from build123d import *

# Parameters (mm, degrees)
F0_R     = 3.81
F1_DEPTH = 25.4


with BuildPart() as f1:
    # F0 (on Top) → F1 (new body)
    with BuildSketch(Plane.XY):
        Polygon((-116.922736, 72.318586), (-370.922736, 72.318586), (-370.922736, 46.918586), (-256.622736, 48.152742), (-256.622736, 35.452742), (-243.922736, 35.452742), (-243.922736, 48.152742), (-129.622736, 48.152742), (-129.622736, 35.452742), (-116.922736, 35.452742), (-116.922736, 46.918586), align=None)
        with Locations((-250.272736, 41.802742)):
            Circle(F0_R, mode=Mode.SUBTRACT)
        with Locations((-122.94844, 41.478446)):
            Circle(F0_R, mode=Mode.SUBTRACT)
    extrude(amount=F1_DEPTH)


solid = f1.part
Can you work these out from the model? Positions are in its coordinate system, mm. A direction names the side the tool comes from. Coordinates: 2 decimals unless noted, no trailing zeros. Write each loop counter-clockwise with the first axis right and the second up, starting at its lowest first coordinate (ties: lowest second). Pieces come first, ordered by that corner, then holes. Notation, with made-up numbers: (74.5, -27.5) - (103.5, -27.5) arc R16 cw to (103.5, -13.5) - close; hole circle Ø3 at (60.25, -40). An arc over 180 degrees is marked (long way). Return JSON: item names as keys, results as strings. Group by question number.
Item 1: I'm going to push a flat-ended pin straight in: pin 1 Ø6.5 at (y, z) = (39, 13) entering from -X. Where does the tip first touch, or does it pass through?
Item 2: If we section it at C-C (x = -352.5): Write out the boundary of the cut face in (y, z).
Item 3: Please list where these lines run through material, in increasing order: probe 1 along X at (y, z) = (42, 15); probe 2 along X at (y, z) = (46, 23); probe 3 along Y at (x, z) = (-171, 19.25).
Item 4: If we section it at B-B (x = -137.5): Write out the boundary of the cut face in (y, z).
Item 5: We'd pull the mould along X, two halves only. Please class faces 1 (the face through (-129.623, 42, 13)), 2 (the face through (-116.923, 54, 13)), 3 (the face through (-242, 72.319, 13)): pulls with the +X half, pulls with the -X half, needs draft (parallel to the pull), parting line crosses it, or undercut.
Item 6: Which directions (+Z, -Z, +X, -X, +Y, -Y) give clear straight access to the entire face, cutting with the end or side of a thin tool? Please do faces 4 (the face through (-188, 48.153, 13)), 5 (the face through (-253.08, 44.38, 12.52)).
Item 7: If we section it at A-A (z = 22): Write out the boundary of the cut face in (x, y).
Return value:
{
 "1": {"pin 1": "stops at x = -256.62"},
 "2": {"outline": "(47.12, 0) - (72.32, 0) - (72.32, 25.4) - (47.12, 25.4) - close"},
 "3": {"probe 1": "x = -256.62 to -254.08, -246.47 to -243.92, -129.62 to -126.72, -119.17 to -116.92", "probe 2": "x = -256.62 to -243.92, -129.62 to -116.92", "probe 3": "y = 48.15 to 72.32"},
 "4": {"outline": "(48.15, 0) - (72.32, 0) - (72.32, 25.4) - (48.15, 25.4) - close"},
 "5": {"face 1": "undercut", "face 2": "pulls with the +X half", "face 3": "needs draft"},
 "6": {"face 4": "+Z, -Z, -Y", "face 5": "+Z, -Z"},
 "7": {"outline": "(-370.92, 46.92) - (-256.62, 48.15) - (-256.62, 35.45) - (-243.92, 35.45) - (-243.92, 48.15) - (-129.62, 48.15) - (-129.62, 35.45) - (-116.92, 35.45) - (-116.92, 72.32) - (-370.92, 72.32) - close; hole circle Ø7.62 at (-250.27, 41.8); hole circle Ø7.62 at (-122.95, 41.48)"}
}
